Input: dimensioned drawing with shaded views. Units: mm. Origin: part minimum x, y, z. A direction names the side the tool comes from. Coordinates: 2 decimals unless noted, no trailing zeros. Order: outer loops, then holes, each group sorted by start corner. A loop starts at its lowest first (then second) coordinate and runs counter-clockwise, first axis right, second up. Notation, with made-up numbers: (13, 62) - (49, 62) arc R28 ccw to (49, 83) - close; hole circle Ø7 at (-33, 75.5). An arc over 180 degrees is marked (long way). One line per question, with ' | ' between items. Start each with the question number.
(1) Section C-C (y = 11.75). Return the cut outline in (x, z), then the cut area to 3 significant figures.
(2) Access query for the marked faces 1 and 2. Directions: +Z, -Z, +X, -X, +Y, -Y. A direction counts if a zero-diameter tool reaches every point of the face in a straight line with its end or side. Return the directions, or none.
(3) Draft query along Y for the marked faces 3, 4 and 5. Return one class per face: +Y half, -Y half, draft (parallel to the pull), parting line (faces both ways), or undercut.
(4) Section B-B (z = 1.5). Return the cut outline in (x, y).
(5) Contact query for flat-ended pins moving along their axis: P1, Ø3, axis at x = 6.5, z = 4, coming from the +Y side; P2, Ø1, axis at x = 15, z = 4, coming from the +Y side; P3, Ø1.5, axis at y = 7.5, z = 1, coming from the +X side. Output: stop coordinate, or through.
(6) Section A-A (x = 4.75). Return the cut outline in (y, z).
(7) Line query: line 1 along Y through (x, z) = (7, 0.5); line 2 along Y through (x, z) = (11.25, 6.25); line 3 along X through (y, z) = (13.5, 3.75) (1 decimal). Output: solid intervals per line, ascending.
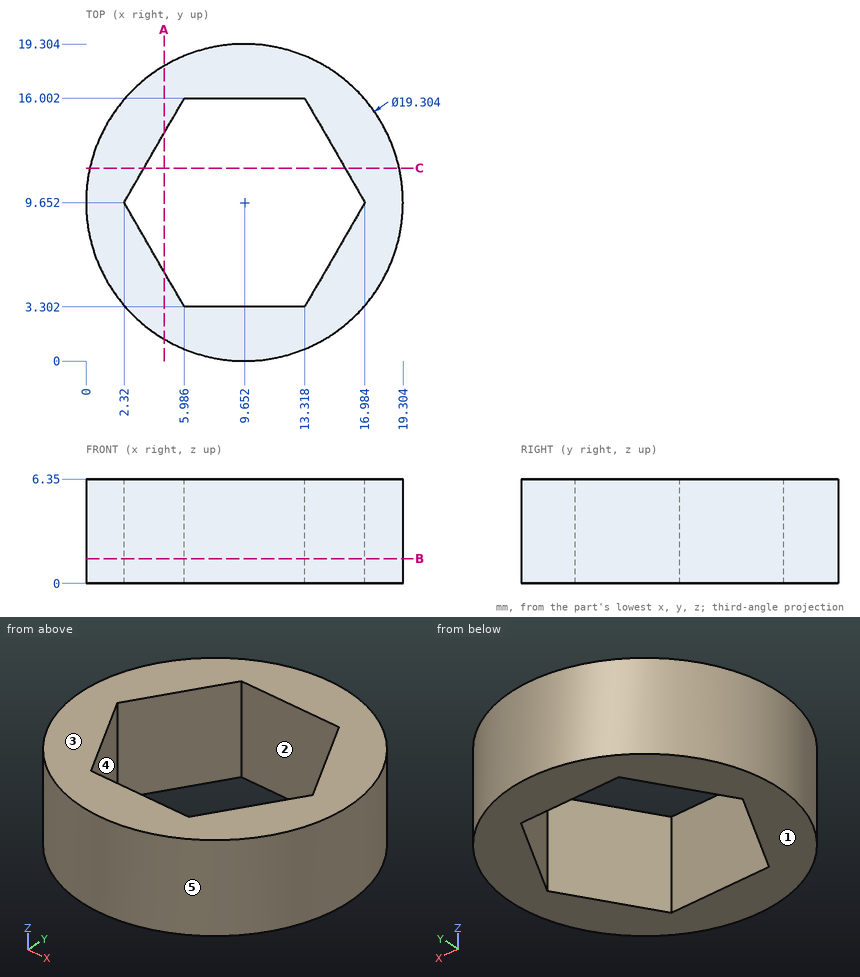
Response values:
1) outline: (0.23, 0) - (3.53, 0) - (3.53, 6.35) - (0.23, 6.35) - close; (15.77, 0) - (19.07, 0) - (19.07, 6.35) - (15.77, 6.35) - close | area: 41.9 mm²
2) face 1: -Z, +X, -X, +Y, -Y | face 2: +Z, -Z
3) face 3: draft | face 4: undercut | face 5: parting line
4) outline: circle Ø19.3 at (9.65, 9.65); hole (2.32, 9.65) - (5.99, 3.3) - (13.32, 3.3) - (16.98, 9.65) - (13.32, 16) - (5.99, 16) - close
5) P1: stops at y = 19.16 | P2: stops at y = 18 | P3: stops at x = 19.2
6) outline: (1.34, 0) - (5.44, 0) - (5.44, 6.35) - (1.34, 6.35) - close; (13.86, 0) - (17.97, 0) - (17.97, 6.35) - (13.86, 6.35) - close
7) line 1: y = 0.37 to 3.3, 16 to 18.93 | line 2: y = 0.13 to 3.3, 16 to 19.17 | line 3: x = 0.8 to 4.5, 14.8 to 18.5
